Source: CAD feature listing. Evaluate the final solid. Frame: model axes, mm. A direction names the side the tool comes from. Give positions to 0.01 mm unless a question says otherwise; leave off trailing zeros. Order: outer loops, then holes, each group sorted by start corner. A loop starts at its lowest first (then second) coordinate and runs counter-clockwise, first axis right, second up.
from build123d import *

# Parameters (mm, degrees)
SKETCH1_W           = 482.6
SKETCH1_H           = 304.8
SKETCH1_R           = 2.5019
BOSS_EXTRUDE1_DEPTH = 12.7
BOSS_EXTRUDE2_DEPTH = 6.35
SKETCH4_W           = 6.35
SKETCH4_H           = 12.7
BOSS_EXTRUDE3_DEPTH = 292.1
SKETCH5_W           = 12.7
SKETCH5_H           = 19.05
BOSS_EXTRUDE4_DEPTH = 6.35
CUT_EXTRUDE2_START  = 6.35
CUT_EXTRUDE2_DEPTH  = 25.4
CUT_EXTRUDE3_START  = -463.55
CUT_EXTRUDE3_DEPTH  = 25.4
BOSS_EXTRUDE5_START = -2.54
BOSS_EXTRUDE5_DEPTH = 7.62
SKETCH13_W          = 152.4
SKETCH13_H          = 27.7368
CUT_EXTRUDE4_DEPTH  = 5.588
SKETCH14_W          = 7.62
SKETCH14_H          = 19.05
CUT_EXTRUDE5_DEPTH  = 12.7


with BuildPart() as part:
    # Sketch1 → Boss-Extrude1 (new body)
    with BuildSketch(Plane(origin=(0, 0, 0), x_dir=(1, 0, 0), z_dir=(0, 1, 0))):
        Rectangle(SKETCH1_W, SKETCH1_H)
        with Locations(Location((-203.2, -135.8392, 0), (0, 0, 270))):
            Circle(SKETCH1_R, mode=Mode.SUBTRACT)
        with Locations(Location((-139.7, -135.8392, 0), (0, 0, 270))):
            Circle(SKETCH1_R, mode=Mode.SUBTRACT)
        with Locations(Location((-76.2, -135.8392, 0), (0, 0, 270))):
            Circle(SKETCH1_R, mode=Mode.SUBTRACT)
        with Locations(Location((88.9, -135.8392, 0), (0, 0, 270))):
            Circle(SKETCH1_R, mode=Mode.SUBTRACT)
        with Locations(Location((152.4, -135.8392, 0), (0, 0, 270))):
            Circle(SKETCH1_R, mode=Mode.SUBTRACT)
        with Locations(Location((215.9, -135.8392, 0), (0, 0, 270))):
            Circle(SKETCH1_R, mode=Mode.SUBTRACT)
    extrude(amount=BOSS_EXTRUDE1_DEPTH)

    # Sketch2 → Boss-Extrude2 (add)
    with BuildSketch(Plane(origin=(0, 12.7, 0), x_dir=(1, 0, 0), z_dir=(0, 1, 0))):
        Polygon((-241.3, 152.4), (-228.6, 152.4), (228.6, 152.4), (241.3, 152.4), (241.3, -152.4), (228.6, -152.4), (228.6, 28.575), (-228.6, 28.575), (-228.6, -152.4), (-241.3, -152.4), align=None)
    extrude(amount=BOSS_EXTRUDE2_DEPTH)

    # Sketch4 → Boss-Extrude3 (add)
    with BuildSketch(Plane.XY.offset(152.4)):
        with Locations((-244.475, 6.35)):
            Rectangle(SKETCH4_W, SKETCH4_H)
    boss_extrude3 = extrude(amount=-BOSS_EXTRUDE3_DEPTH)

    # Sketch5 → Boss-Extrude4 (add)
    with BuildSketch(Plane.ZY.offset(241.3)):
        with Locations((-146.05, 9.525)):
            Rectangle(SKETCH5_W, SKETCH5_H)
    boss_extrude4 = extrude(amount=BOSS_EXTRUDE4_DEPTH)

    # Mirror1: Boss-Extrude3, Boss-Extrude4 across plane
    add(boss_extrude3.mirror(Plane(origin=(0, 0, 0), x_dir=(0, 0, 1), z_dir=(1, 0, 0))))
    add(boss_extrude4.mirror(Plane(origin=(0, 0, 0), x_dir=(0, 0, 1), z_dir=(1, 0, 0))))

    # Sketch6 → Cut-Extrude2 (cut)
    with BuildSketch(Plane.ZY.offset(241.3).offset(CUT_EXTRUDE2_START)):
        with BuildLine():
            Line((147.32, 2.54), (128.27, 2.54))
            ThreePointArc((128.27, 2.54), (124.46, 6.35), (128.27, 10.16))
            Line((128.27, 10.16), (147.32, 10.16))
            ThreePointArc((147.32, 10.16), (151.13, 6.35), (147.32, 2.54))
        make_face()
    extrude(amount=-CUT_EXTRUDE2_DEPTH, mode=Mode.SUBTRACT)

    # Sketch6<2> → Cut-Extrude3 (cut)
    with BuildSketch(Plane.ZY.offset(241.3).offset(CUT_EXTRUDE3_START)):
        with BuildLine():
            Line((147.32, 2.54), (128.27, 2.54))
            ThreePointArc((128.27, 2.54), (124.46, 6.35), (128.27, 10.16))
            Line((128.27, 10.16), (147.32, 10.16))
            ThreePointArc((147.32, 10.16), (151.13, 6.35), (147.32, 2.54))
        make_face()
    extrude(amount=-CUT_EXTRUDE3_DEPTH, mode=Mode.SUBTRACT)

    # Sketch11 → Boss-Extrude5 (add)
    with BuildSketch(Plane.XZ.offset(BOSS_EXTRUDE5_START)):
        Polygon((-247.65, 124.46), (-222.25, 124.46), (-222.25, 140.97), align=None)
    boss_extrude5 = extrude(amount=-BOSS_EXTRUDE5_DEPTH)

    # Mirror2: Boss-Extrude5 across plane
    add(boss_extrude5.mirror(Plane(origin=(0, 0, 0), x_dir=(0, 0, 1), z_dir=(1, 0, 0))))

    # Sketch13 → Cut-Extrude4 (cut)
    with BuildSketch(Plane(origin=(0, 12.7, 0), x_dir=(1, 0, 0), z_dir=(0, 1, 0))):
        with Locations((146.05, -138.5316)):
            Rectangle(SKETCH13_W, SKETCH13_H)
        with Locations((-146.05, -138.5316)):
            Rectangle(SKETCH13_W, SKETCH13_H)
    extrude(amount=-CUT_EXTRUDE4_DEPTH, mode=Mode.SUBTRACT)

    # Sketch14 → Cut-Extrude5 (cut)
    with BuildSketch(Plane.XZ):
        with Locations((43.18, -29.845)):
            Rectangle(SKETCH14_W, SKETCH14_H)
    extrude(amount=-CUT_EXTRUDE5_DEPTH, mode=Mode.SUBTRACT)


solid = part.part
1) Ray query, L1, parallel to X at y = 11, z = -26.5; L2, parallel to X at y = 15.5, z = 77; L3, parallel to Z at x = 105, y = 15.75 (3 decimals). Return the intervals inside material, ascending.
Checks:
L1: x = -247.65 to 39.37, 46.99 to 247.65
L2: x = -241.3 to -228.6, 228.6 to 241.3
L3: z = -152.4 to -28.575
2) Section query A-A on x = -149.5. Output: boundary loops of the cut face in (y, z) (3 decimals).
Checks:
outline: (0, -152.4) - (19.05, -152.4) - (19.05, -28.575) - (12.7, -28.575) - (12.7, 124.663) - (7.112, 124.663) - (7.112, 152.4) - (0, 152.4) - close
3) Reachability of faces 4 (the face through (-147, 7.112, 138)), 5 (the face through (-3, 9, -152.4)), 6 (the face through (234.77, 6.3, 132.83)), 7 (the face through (-238, 2.54, 140)), 8 (the face through (39.37, 6, -30)) from +Z, -Z, +X, -X, +Y, -Y: full face, straight path, thin tool, end or side. Return the list, or none.
Checks:
face 4: +Z, +Y
face 5: -Z, +X, -X, +Y, -Y
face 6: +X
face 7: -X
face 8: -Y
4) Section query B-B on z = 79.5. Output: boundary loops of the cut face in (x, y).
Checks:
outline: (-247.65, 0) - (247.65, 0) - (247.65, 12.7) - (241.3, 12.7) - (241.3, 19.05) - (228.6, 19.05) - (228.6, 12.7) - (-228.6, 12.7) - (-228.6, 19.05) - (-241.3, 19.05) - (-241.3, 12.7) - (-247.65, 12.7) - close
5) First-contact query: pin 1 Ø1.9 at (y, z) = (15, 38) entering from +X; pin 2 Ø5 at (x, z) = (130.5, 5) entering from +Y; pin 3 Ø8 at (x, z) = (-203.2, 135.84) entering from +Y. Flat tips, straight axial feed; report the tip coordinate or a pass-through.
Checks:
pin 1: stops at x = 241.3
pin 2: stops at y = 12.7
pin 3: stops at y = 7.11
6) Pull-direction query (X, two-part tool) for faces 1 (the face through (46.99, 6, -30)), 2 (the face through (-238, 10.16, 140)), 3 (the face through (-234.77, 6.3, 132.83)); classes: +X half, -X half, draft (parallel to the pull), parting line (faces both ways), or undercut.
Checks:
face 1: undercut
face 2: draft
face 3: -X half
